The model under review builds one solid part; all positions refer to its coordinate system, in mm. Face numbers are marked on the shaded views. A direction names the side the tool comes from. Coordinates: 2 decimals unless noted, no trailing zeros. Order: outer loops, then holes, each group sorted by start corner. A loop starts at its lowest first (then second) coordinate and runs counter-clockwise, first axis right, second up. Notation, with made-up numbers: (20.25, 77.25) -> (32.25, 77.25) arc R33 cw to (32.25, 107.25) -> close; hole circle Ø4 at (85, 4.25). An arc over 180 degrees is marked (long way). Use one line per item in the form item = value. Start each with the question number.
(1) For the marked faces 1 and 2, list the 3-axis set-ups (+Z, -Z, +X, -X, +Y, -Y) from which the entire face can be reached by the end or side of a thin tool; tool diameter is ignored.
(2) Take a section at C-C (y = 10). State the section outline as (x, z) points.
(3) Take a section at D-D (x = -6). State the section outline as (y, z) points.
(4) Wall thickness on line 1 along Z through (x, y) = (-20, 1.45); line 2 along Y through (x, z) = (-10, -38): over which ranges is each line inside the solid? List them lowest first.
(5) Take a section at B-B (x = -30). State how many separate pieces and enclosed holes the cut face has, then the cut area to 3 significant figures.
(6) Insertion check: pin 1 Ø4 at (x, y) = (-20, 10) entering from +Z; pin 2 Ø6 at (x, y) = (-22, 24) entering from +Z; pin 3 Ø7 at (x, z) = (-10, -20) entering from +Y. Each pin has a flat end and moves straight along its axis. Give the tip position at first contact, or say it passes through.
(7) Take a section at A-A (z = -10). State the section outline as (x, y) points.
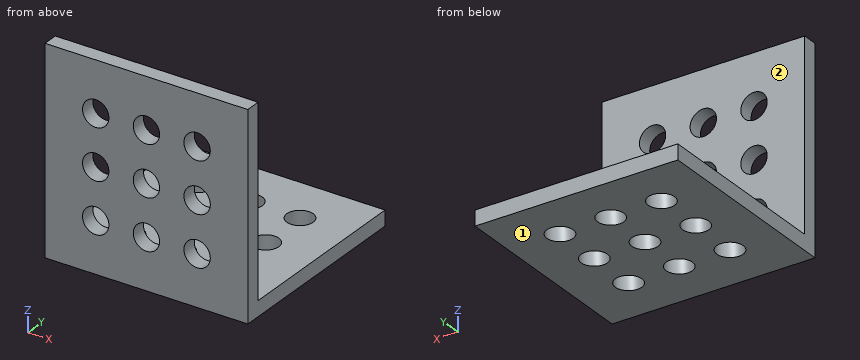
```python
from build123d import *

# Parameters (mm, degrees)
BOSS_EXTRUDE1_DEPTH = 40
SKETCH2_R           = 2.6
CUT_EXTRUDE1_DEPTH  = 4


with BuildPart() as part:
    # Sketch1 → Boss-Extrude1 (new body)
    with BuildSketch(Plane(origin=(0, 0, 0), x_dir=(0, 0, -1), z_dir=(1, 0, 0))):
        Polygon((0, 0), (0, 3), (37, 3), (37, 40), (40, 40), (40, 0), align=None)
    extrude(amount=-BOSS_EXTRUDE1_DEPTH)

    # Sketch2 → Cut-Extrude1 (cut, through all)
    with BuildSketch(Plane(origin=(0, 3, 0), x_dir=(1, 0, 0), z_dir=(0, 1, 0))):
        with Locations((-30, 10)):
            Circle(SKETCH2_R)
        with Locations((-20, 10)):
            Circle(SKETCH2_R)
        with Locations((-10, 10)):
            Circle(SKETCH2_R)
        with Locations((-20, 20)):
            Circle(SKETCH2_R)
        with Locations((-10, 20)):
            Circle(SKETCH2_R)
        with Locations((-20, 30)):
            Circle(SKETCH2_R)
        with Locations((-10, 30)):
            Circle(SKETCH2_R)
        with Locations((-30, 20)):
            Circle(SKETCH2_R)
        with Locations((-30, 30)):
            Circle(SKETCH2_R)
    cut_extrude1 = extrude(amount=-CUT_EXTRUDE1_DEPTH, mode=Mode.SUBTRACT)

    # Mirror1: Cut-Extrude1 across plane
    add(cut_extrude1.mirror(Plane(origin=(0, 20, -20), x_dir=(0, 0.707106781, 0.707106781), z_dir=(0, 0.707106781, -0.707106781))), mode=Mode.SUBTRACT)


solid = part.part
```
Findings:
q1.face_1 = -Z, +X, -X, +Y, -Y
q1.face_2 = +Z, +X, -X, +Y
q2.outline = (-40, -40) -> (-32.6, -40) -> (-32.6, -37) -> (-40, -37) -> close; (-27.4, -40) -> (-22.6, -40) -> (-22.6, -37) -> (-27.4, -37) -> close; (-17.4, -40) -> (-12.6, -40) -> (-12.6, -37) -> (-17.4, -37) -> close; (-7.4, -40) -> (0, -40) -> (0, -37) -> (-7.4, -37) -> close
q3.outline = (0, -40) -> (40, -40) -> (40, -37) -> (3, -37) -> (3, 0) -> (0, 0) -> close
q4.line_1 = -40 to -32.6, -27.4 to -22.6, -17.4 to -12.6, -7.4 to 0
q4.line_2 = 0 to 7.4, 12.6 to 17.4, 22.6 to 27.4, 32.6 to 40
q5.separate_pieces = 7
q5.enclosed_holes = 0
q5.area = 137 mm²
q6.pin_1 = through
q6.pin_2 = -37
q6.pin_3 = 3
q7.outline = (-40, 0) -> (-32.6, 0) -> (-32.6, 3) -> (-40, 3) -> close; (-27.4, 0) -> (-22.6, 0) -> (-22.6, 3) -> (-27.4, 3) -> close; (-17.4, 0) -> (-12.6, 0) -> (-12.6, 3) -> (-17.4, 3) -> close; (-7.4, 0) -> (0, 0) -> (0, 3) -> (-7.4, 3) -> close
